Part model, mm, in its own coordinate system. A direction names the side the tool comes from. Give positions to 0.01 mm unless a question says otherwise; leave off trailing zeros. Order: outer loops, then holes, each group sorted by start corner. A loop starts at its lowest first (then second) coordinate and runs counter-clockwise, first axis right, second up. Notation, with made-up numbers: M -17,5.5 L 24,5.5 A17 cw 24,9.5 Z; hole C -15,11 d3. An arc over 180 degrees is marked long. Return JSON: item names as keys, results as strings.
from build123d import *

# Parameters (mm, degrees)
F1_DEPTH  = 130
F4_DEPTH  = 121
F6_DEPTH  = 116
F8_W      = 5
F8_H      = 55
F9_DEPTH  = 37.8
F10_W     = 5
F10_H     = 55
F11_DEPTH = 63
F12_R     = 5
F13_DEPTH = 135
F14_R     = 6
F15_DEPTH = 25


with BuildPart() as f1:
    # F0 (on Top) → F1 (new body)
    with BuildSketch(Plane.XY):
        with BuildLine():
            Line((69, 0), (0, 0))
            Line((0, 0), (0, -5))
            Line((0, -5), (69, -5))
            ThreePointArc((69, -5), (71.1213203436, -5.8786796564), (72, -8))
            Line((72, -8), (72, -103))
            ThreePointArc((72, -103), (71.1213203436, -105.1213203436), (69, -106))
            Line((69, -106), (0, -106))
            Line((0, -106), (0, -111))
            Line((0, -111), (69, -111))
            ThreePointArc((69, -111), (74.6568542495, -108.6568542495), (77, -103))
            Line((77, -103), (77, -8))
            ThreePointArc((77, -8), (74.6568542495, -2.3431457505), (69, 0))
        make_face()
    extrude(amount=F1_DEPTH)

    # F3 (on offset) → F4 (cut)
    with BuildSketch(Plane(origin=(0, 0, 0), x_dir=(-1, 0, 0), z_dir=(0, 1, 0))):
        Polygon((0, 75), (0, 130), (-72, 130), (-72, 75), (-42, 75), align=None)
    extrude(amount=-F4_DEPTH, mode=Mode.SUBTRACT)

    # F5 (on offset) → F6 (cut)
    with BuildSketch(Plane(origin=(0, 0, 0), x_dir=(-1, 0, 0), z_dir=(0, 1, 0))):
        Polygon((0, 30), (0, 75), (-42, 75), align=None)
    extrude(amount=-F6_DEPTH, mode=Mode.SUBTRACT)

    # F8 (on offset) → F9 (cut)
    with BuildSketch(Plane.YZ.offset(77)):
        with Locations((-2.5, 102.5)):
            Rectangle(F8_W, F8_H)
    extrude(amount=-F9_DEPTH, mode=Mode.SUBTRACT)

    # F10 (on offset) → F11 (cut)
    with BuildSketch(Plane.YZ.offset(77)):
        with Locations((-108.5, 102.5)):
            Rectangle(F10_W, F10_H)
    extrude(amount=-F11_DEPTH, mode=Mode.SUBTRACT)

    # F12 (on offset) → F13 (cut)
    with BuildSketch(Plane(origin=(0, 0, 0), x_dir=(-1, 0, 0), z_dir=(0, 1, 0))):
        with Locations((-15, 25)):
            Circle(F12_R)
        with Locations((-50, 25)):
            Circle(F12_R)
    extrude(amount=-F13_DEPTH, mode=Mode.SUBTRACT)

    # F14 (on offset) → F15 (cut)
    with BuildSketch(Plane.YZ.offset(77)):
        with Locations((-55.5, 25)):
            Circle(F14_R)
        with Locations((-77, 105)):
            Circle(F14_R)
        with Locations((-34, 105)):
            Circle(F14_R)
    extrude(amount=-F15_DEPTH, mode=Mode.SUBTRACT)


solid = f1.part
Q1. Band-saw the part on D-D (z = 105). Give the cut face in (x, y).
Established:
{"outline": "M 72,-106 L 76.42,-106 A8 ccw 77,-103 L 77,-83 L 72,-83 Z; M 72,-71 L 77,-71 L 77,-40 L 72,-40 Z; M 72,-28 L 77,-28 L 77,-8 A8 ccw 76.42,-5 L 72,-5 Z"}
Q2. Band-saw the part on A-A (x = 53). Give the cut face in (y, z), then the cut area to 3 significant figures.
Established:
{"outline": "M -111,0 L -106,0 L -106,21 L -111,21 Z; M -111,29 L -106,29 L -106,75 L -111,75 Z; M -5,0 L 0,0 L 0,21 L -5,21 Z; M -5,29 L 0,29 L 0,75 L -5,75 Z", "area": "670 mm²"}
Q3. Band-saw the part on C-C (z = 25). Give the number of separate pieces and of enclosed holes in the cut face, then the cut area to 3 significant figures.
Established:
{"separate pieces": "6", "enclosed holes": "0", "area": "991 mm²"}
Q4. 3-axis set-ups, long thin cutter, end or side, ignore diameter. For faces 1 (the flat face through (42, -5, 29)), 2 (the cylindrical face through (74.54, -81.42, 109.06)): which of +Z, -Z, +X, -X, +Y, -Y reach the whole face in a straight line?
Established:
{"face 1": "+Z, -Z, -X", "face 2": "+X, -X"}
Q5. Pin check, flat tips, straight feed: pin 1 (14 mm diameter, centred on y = -77, z = 105, fed in from -X); pin 2 (2 mm diameter, centred on x = 74, z = 91.5, fed in from -Y); pin 3 (2.5 mm diameter, centred on x = 59.5, y = -3, fed in from +Z). Stop position of each tip, or through.
Established:
{"pin 1": "stops at x = 72", "pin 2": "stops at y = -106", "pin 3": "stops at z = 75"}
Q6. Probe line 1 along Y through (x, z) = (28, 30); line 2 along Z through (x, y) = (74.5, -34); line 3 along X through (y, z) = (-98, 96). List the from-to ranges inside material, lowest first.
Established:
{"line 1": "y = -111 to -106, -5 to 0", "line 2": "z = 0 to 99, 111 to 130", "line 3": "x = 72 to 77"}
Q7. Band-saw the part on B-B (y = -77). Give the cut face in (x, z), then the cut area to 3 significant figures.
Established:
{"outline": "M 72,0 L 77,0 L 77,99 L 72,99 Z; M 72,111 L 77,111 L 77,130 L 72,130 Z", "area": "590 mm²"}
Q8. Two-plate mould, pull along Z, no slides. Class faces 3 (the cylindrical face through (74.54, -34.78, 110.95)), 4 (the flat face through (21.294, -108.465, 52.815)), 5 (the cylindrical face through (71.14, -105.1, 36.98)): +Z half, -Z half, draft (parallel to the pull), parting line (faces both ways), or undercut.
Established:
{"face 3": "undercut", "face 4": "+Z half", "face 5": "draft"}
